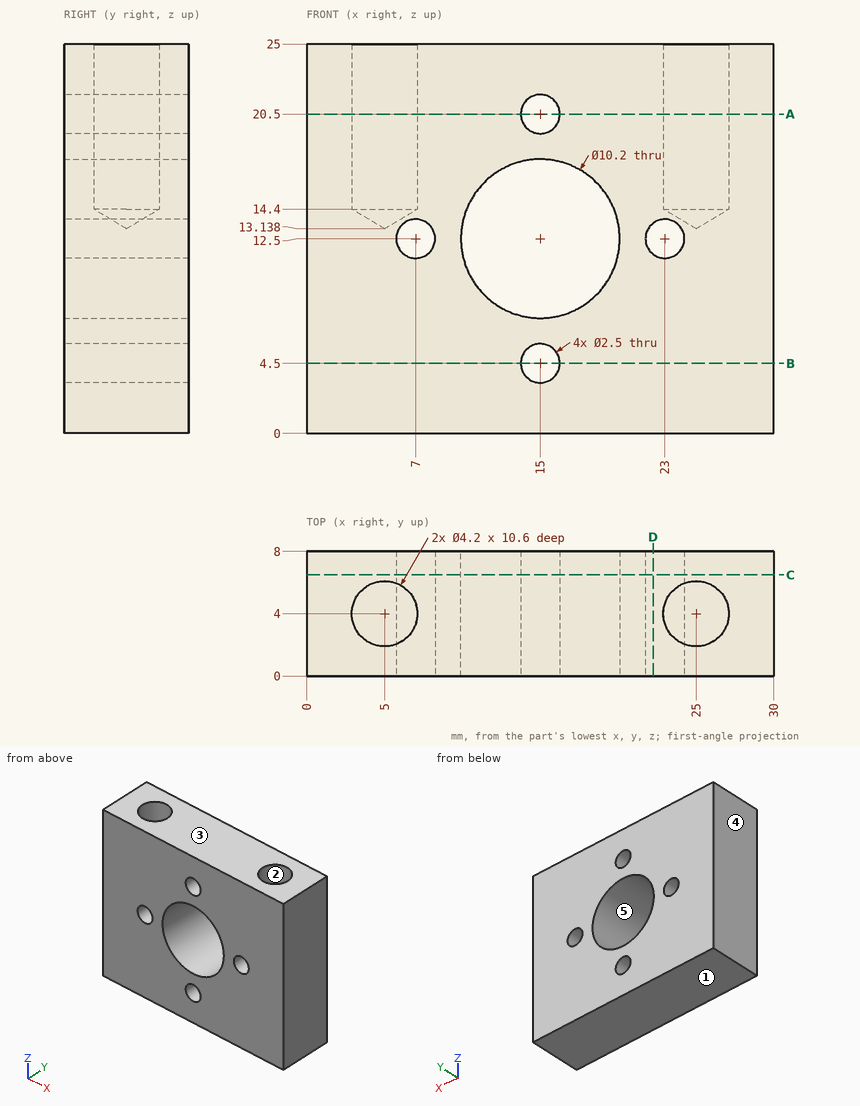
Verification items for this drawing (mm, ordinates from the low corner). A direction names the side the tool comes from. Round coordinates to 2 decimals unless told otherwise and drop trailing zeros. Order: outer loops, then holes, each group sorted by start corner. A loop starts at its lowest first (then second) coordinate and runs counter-clockwise, first axis right, second up. Notation, with made-up numbers: (-32, 52.25) - (26, 52.25) arc R27 cw to (26, 83.25) - close; hole circle Ø1 at (84, 23). An arc over 180 degrees is marked (long way). Use CSV: the item, a comma, the result in double quotes. Start each with the question number.
1) Go/stop test with flat-tipped pins: P1, Ø2, axis at x = 23, z = 12.5, coming from the +Y side; P2, Ø3.5, axis at x = 25, y = 4, coming from the +Z side. Record where each tip stops, or that it passes through.
2) Section check D-D, the plane x = 22.25. Record the cut outline in (y, z), plus the area to 3 significant figures.
3) Section check C-C, the plane y = 6.5. Record the cut outline in (x, z).
4) Section check A-A, the plane z = 20.5. Record the cut outline in (x, y), plus the area to 3 significant figures.
5) Access from +Z, -Z, +X, -X, +Y, -Y to the whole of each face (thin tool, end or side, straight path). Record for the marked faces 1 and 2.
6) Mould release check, pull along X, two halves, no side actions. Record for the marked faces 3, 4 and 5: +X half, -X half, draft (parallel to the pull), parting line (faces both ways), or undercut.
7) Thickness scan on L1, parallel to Z at x = 15, y = 4.25; L2, parallel to X at y = 1.5, z = 11.75 (1 decimal); L3, parallel to X at y = 4, z = 19.5. Record the ranges inside material, lowest first.
8) Section check B-B, the plane z = 4.5. Record the cut outline in (x, y), plus the area to 3 significant figures.
Answers:
1,P1,"passes through"
1,P2,"stops at z = 14.19"
2,outline,"(0, 0) - (8, 0) - (8, 11.5) - (0, 11.5) - close; (0, 13.5) - (8, 13.5) - (8, 25) - (0, 25) - close"
2,area,"184 mm²"
3,outline,"(0, 0) - (30, 0) - (30, 25) - (0, 25) - close; hole circle Ø2.5 at (7, 12.5); hole circle Ø10.2 at (15, 12.5); hole circle Ø2.5 at (15, 4.5); hole circle Ø2.5 at (15, 20.5); hole circle Ø2.5 at (23, 12.5)"
4,outline,"(0, 0) - (13.75, 0) - (13.75, 8) - (0, 8) - close; (16.25, 0) - (30, 0) - (30, 8) - (16.25, 8) - close; hole circle Ø4.2 at (5, 4); hole circle Ø4.2 at (25, 4)"
4,area,"192 mm²"
5,face 1,"-Z, +X, -X, +Y, -Y"
5,face 2,"+Z"
6,face 3,"draft"
6,face 4,"-X half"
6,face 5,"undercut"
7,L1,"z = 0 to 3.25, 5.75 to 7.4, 17.6 to 19.25, 21.75 to 25"
7,L2,"x = 0 to 6, 8 to 10, 20 to 22, 24 to 30"
7,L3,"x = 0 to 2.9, 7.1 to 14.25, 15.75 to 22.9, 27.1 to 30"
8,outline,"(0, 0) - (13.75, 0) - (13.75, 8) - (0, 8) - close; (16.25, 0) - (30, 0) - (30, 8) - (16.25, 8) - close"
8,area,"220 mm²"
